from build123d import *

# Parameters (mm, degrees)
CROQUIS1_R              = 112.5
SALIENTE_EXTRUIR1_DEPTH = 10
MATRIZC1_COUNT          = 6
CROQUIS6_R              = 90
SALIENTE_EXTRUIR2_DEPTH = 4


with BuildPart() as part:
    # Croquis1 → Saliente-Extruir1 (new body)
    with BuildSketch(Plane(origin=(0, 0, 0), x_dir=(1, 0, 0), z_dir=(0, 1, 0))):
        with Locations(Location((0, 0, 0), (0, 0, 270))):
            Circle(CROQUIS1_R)
    extrude(amount=SALIENTE_EXTRUIR1_DEPTH)

    # Croquis5 → Taladro de margen para M121 (revolve, cut)
    with BuildSketch(Plane(origin=(0, 10, -102.5), x_dir=(0, 0, 1), z_dir=(1, 0, 0))):
        Polygon((0, 0), (0, 47.555809178), (6.75, 43.5), (6.75, 0), align=None)
    taladro_de_margen_para_m121 = revolve(axis=Axis((0, 16.35, -102.5), (0, -1, 0)), mode=Mode.SUBTRACT)

    # MatrizC1: Taladro de margen para M121 ×6 about axis
    matrizc1_axis = Axis((0, 0, 0.3703332), (0, 1, 0))
    for i in range(1, MATRIZC1_COUNT):
        add(taladro_de_margen_para_m121.rotate(matrizc1_axis, i * 360 / MATRIZC1_COUNT), mode=Mode.SUBTRACT)

    # Croquis6 → Saliente-Extruir2 (add)
    with BuildSketch(Plane(origin=(0, 10, 0), x_dir=(1, 0, 0), z_dir=(0, 1, 0))):
        with Locations(Location((0, 0, 0), (0, 0, 270))):
            Circle(CROQUIS6_R)
    extrude(amount=SALIENTE_EXTRUIR2_DEPTH)


solid = part.part
Read the model definition and answer for the solid it produces. Units are mm, in the model's axes. A direction names the side the tool comes from. Coordinates: 2 decimals unless noted, no trailing zeros. Order: outer loops, then holes, each group sorted by start corner. A loop starts at its lowest first (then second) coordinate and runs counter-clockwise, first axis right, second up. Notation, with made-up numbers: M 15.5,30.5 L 67.5,30.5 A23 cw 67.5,68.5 Z; hole C 73.5,24 d11. An arc over 180 degrees is marked long. Put each result on its own line as item: value. Start each with the question number.
Item 1: The mould has two halves that part along Z. Classify faces 3 (the face through (4.95, 4.93, -112.39)), 4 (the face through (2, 0, -2)), 5 (the face through (-89.385, 5.07, 45.062)): +Z half, -Z half, draft (parallel to the pull), parting line (faces both ways), or undercut.
Item 2: Section D-D, the plane x = 70 is taken. Determine the outline of the cut face in (y, z), plus the area to 3 significant figures.
Item 3: Given pin 1 Ø4 at (x, y) = (34.5, 12.5) entering from -Z; pin 2 Ø21.5 at (x, z) = (89.09, -51.06) entering from +Y; pin 3 Ø6 at (x, y) = (74, 10.5) entering from -Z, each flat-ended and moving along its own axis, determine where each tip first touches the part or whether it passes through.
Item 4: Section C-C, the plane z = 53 is taken. Determine the outline of the cut face in (x, y), plus the area to 3 significant figures.
Item 5: For faces 1 (the face through (-34.471, 11.972, 83.137)), 2 (the face through (95.678, 5.07, 50.342)), determine the directions among +Z, -Z, +X, -X, +Y, -Y from which every point of the face is accessible in a straight line to the end or side of a thin tool.
Item 6: Consider probe 1 along X at (y, z) = (2.75, -49.5); probe 2 along Y at (x, z) = (49, -87.5); probe 3 along X at (y, z) = (7, -102.5). Determine where each line is inside the solid, lowest interval first. Write a range as [from, to].
Item 7: Section A-A, the plane x = 0 is taken. Determine the outline of the cut face in (y, z).
Item 8: Section B-B, the plane z = -102.5 is taken. Determine the outline of the cut face in (x, y), plus the area to 3 significant figures.
Computed:
1. face 3: parting line
1. face 4: draft
1. face 5: undercut
2. outline: M 0,-88.07 L 10,-88.07 L 10,-56.57 L 14,-56.57 L 14,56.57 L 10,56.57 L 10,88.07 L 0,88.07 Z
2. area: 2,210 mm2
3. pin 1: stops at z = -83.93
3. pin 2: stops at y = 10
3. pin 3: stops at z = -87.23
4. outline: M -99.23,0 L -95.73,0 L -95.73,10 L -99.23,10 Z; M -82.44,0 L 82.44,0 L 82.44,10 L 72.74,10 L 72.74,14 L -72.74,14 L -72.74,10 L -82.44,10 Z; M 95.73,0 L 99.23,0 L 99.23,10 L 95.73,10 Z
4. area: 2,300 mm2
5. face 1: +Y
5. face 2: +Y, -Y
6. probe 1: x = [-101.02, -95.65], [-82.52, 82.52], [95.65, 101.02]
6. probe 2: y = [0, 10]
6. probe 3: x = [-46.37, -6.75], [6.75, 46.37]
7. outline: M 0,-112.5 L 10,-112.5 L 10,-109.25 L 0,-109.25 Z; M 0,-95.75 L 10,-95.75 L 10,-90 L 14,-90 L 14,90 L 10,90 L 10,96.49 L 0,96.49 Z; M 0,109.99 L 10,109.99 L 10,112.5 L 0,112.5 Z
8. outline: M -46.37,0 L -6.75,0 L -6.75,10 L -46.37,10 Z; M 6.75,0 L 46.37,0 L 46.37,10 L 6.75,10 Z
8. area: 792 mm2
